Part model, mm, in its own coordinate system. Coordinates: 2 decimals unless noted, no trailing zeros. Loops run counter-clockwise (first coordinate to the right, second up) from the corner with the lowest first, then second, coordinate; pieces in that order, holes last. Notation, with made-up numbers: (77, 86.5) -> (88, 86.5) arc R32 cw to (88, 118.5) -> close; hole circle Ø11 at (-33, 6.5). An arc over 180 degrees is marked (long way). Use one line per item in the form item = value. Start each with the question number.
(1) Band-saw the part on B-B on x = 7.59. Give the cut face in (y, z).
(2) Band-saw the part on C-C on z = 4.35. Count the separate pieces of the cut face and the enclosed holes in it, then the cut area to 3 significant figures.
(3) Band-saw the part on A-A on y = 0. Give the cut face in (x, z).
(4) Mould opens along X. For faces 1 (the flat face through (10, -5, 5)), 2 (the cylindrical face through (22.4, -7.1, 2.5)), 3 (the cylindrical face through (7.5, -11.1, 2.5)) say: +X half, -X half, draft (parallel to the pull), parting line (faces both ways), or undercut.
(5) Band-saw the part on D-D on y = -12. Give the cut face in (x, z).
(6) Pin check, flat tips, straight feed: P1, Ø2, axis at x = 11.5, z = 3.5, coming from the +Y side; P2, Ø5.5, axis at x = 0, y = -15.18, coming from the +Z side; P3, Ø2, axis at y = 11, z = 2.5, coming from the +X side; P4, Ø1, axis at x = 15.5, z = 4, coming from the -Y side. Stop position of each tip, or through.
(7) Drill centre lines: L1, parallel to Y at x = -7.59, z = 1.85; L2, parallel to Y at x = -13.5, z = 1.5; L3, parallel to Y at x = -0.5, z = 1.3. Where is each one in solid material? Low to high. Write a range as [from, to].
Autodesk Inventor part; units mm, degrees
ref_plane "YZ Plane" through (0, 0, 0) normal (1, 0, 0) x (0, 1, 0)
ref_plane "XZ Plane" through (0, 0, 0) normal (0, 1, 0) x (-1, 0, 0)
ref_plane "XY Plane" through (0, 0, 0) normal (0, 0, 1) x (1, 0, 0)
sketch "スケッチ1" plane through (0, 0, 0) normal (0, 0, 1) x (1, 0, 0)
  circle A0 centre (0, 0) radius 23.5
  dimension "d0" = 47
extrude "押し出し1" add sketch "スケッチ1" along normal blind 5
sketch "スケッチ2" plane through (0, 0, 5) normal (0, 0, 1) x (1, 0, 0)
  line L0 (0, 0) -> (0, -15.18)
  circle A0 centre (0, 0) radius 15.18
  line L1 (0, 0) -> (7.59, -13.1463)
  point P0 (13.1463, 7.59)
  point P1 (-13.1463, 7.59)
  point P2 (15.18, 0)
  point P3 (7.59, 13.1463)
  point P4 (-7.59, 13.1463)
  point P5 (-15.18, 0)
  point P6 (-7.59, -13.1463)
  dimension "d3" = 30.36
  dimension "d6" = 360
  dimension "d8" = 30
  dimension "d11" = 360
hole "穴1" at (0, -15.18, 5) at (13.1463, 7.59, 5) at (-13.1463, 7.59, 5) at (7.59, -13.1463, 5) at (15.18, 0, 5) at (7.59, 13.1463, 5) at (-7.59, 13.1463, 5) at (-15.18, 0, 5) at (-7.59, -13.1463, 5) direction (0, 0, -1) diameter 4.1 end through all
sketch "スケッチ3" plane through (0, 0, 5) normal (0, 0, 1) x (1, 0, 0)
  circle A0 centre (0, 0) radius 11
  dimension "d20" = 22
extrude "押し出し2" cut sketch "スケッチ3" against normal blind 5
properties part number "base_plate2" material "アルミニウム 6061"
A:
q1.outline = (-22.24, 0) -> (-15.2, 0) -> (-15.2, 5) -> (-22.24, 5) -> close; (-11.1, 0) -> (-7.96, 0) -> (-7.96, 5) -> (-11.1, 5) -> close; (7.96, 0) -> (11.1, 0) -> (11.1, 5) -> (7.96, 5) -> close; (15.2, 0) -> (22.24, 0) -> (22.24, 5) -> (15.2, 5) -> close
q2.separate_pieces = 1
q2.enclosed_holes = 10
q2.area = 1,240 mm²
q3.outline = (-23.5, 0) -> (-17.23, 0) -> (-17.23, 5) -> (-23.5, 5) -> close; (-13.13, 0) -> (-11, 0) -> (-11, 5) -> (-13.13, 5) -> close; (11, 0) -> (13.13, 0) -> (13.13, 5) -> (11, 5) -> close; (17.23, 0) -> (23.5, 0) -> (23.5, 5) -> (17.23, 5) -> close
q4.face_1 = draft
q4.face_2 = parting line
q4.face_3 = undercut
q5.outline = (-20.21, 0) -> (-9.29, 0) -> (-9.29, 5) -> (-20.21, 5) -> close; (-5.89, 0) -> (5.89, 0) -> (5.89, 5) -> (-5.89, 5) -> close; (9.29, 0) -> (20.21, 0) -> (20.21, 5) -> (9.29, 5) -> close
q6.P1 = 21.02
q6.P2 = 5
q6.P3 = 21.27
q6.P4 = -18.09
q7.L1 = [-22.24, -15.2], [-11.1, -7.96], [7.96, 11.1], [15.2, 22.24]
q7.L2 = [-19.24, -1.17], [1.17, 5.57], [9.61, 19.24]
q7.L3 = [-23.49, -17.17], [-13.19, -10.99], [10.99, 23.49]
